from build123d import *

# Parameters (mm, degrees)
SKETCH1_R           = 3.75
SKETCH1_R_2         = 0.65
BOSS_EXTRUDE1_DEPTH = 2.5
CUT_EXTRUDE1_START  = -1.5
SKETCH2_R           = 0.65
CUT_EXTRUDE1_DEPTH  = 1.5
FILLET1_R           = 3
CUT_EXTRUDE3_DEPTH  = 56.730615831
FILLET2_R           = 1.5


with BuildPart() as part:
    # Sketch1 → Boss-Extrude1 (new body)
    with BuildSketch(Plane(origin=(0, 0, 0), x_dir=(1, 0, 0), z_dir=(0, 1, 0))):
        Polygon((0, 0), (0, 12), (50, 25.397459622), (50, 0), align=None)
        with Locations(Location((5.75, 6, 0), (0, 0, 270))):
            Circle(SKETCH1_R, mode=Mode.SUBTRACT)
        with Locations(Location((22.75, 6, 0), (0, 0, 270))):
            Circle(SKETCH1_R_2, mode=Mode.SUBTRACT)
        with Locations(Location((45.166201183, 17.5, 0), (0, 0, 270))):
            Circle(SKETCH1_R, mode=Mode.SUBTRACT)
        with Locations(Location((36.666201183, 2.777568136, 0), (0, 0, 270))):
            Circle(SKETCH1_R_2, mode=Mode.SUBTRACT)
        with Locations(Location((37.916201183, 4.942631645, 0), (0, 0, 270))):
            Circle(SKETCH1_R_2, mode=Mode.SUBTRACT)
        with Locations(Location((39.166201183, 7.107695155, 0), (0, 0, 270))):
            Circle(SKETCH1_R_2, mode=Mode.SUBTRACT)
        with Locations(Location((40.416201183, 9.272758664, 0), (0, 0, 270))):
            Circle(SKETCH1_R_2, mode=Mode.SUBTRACT)
        with Locations(Location((41.666201183, 11.437822174, 0), (0, 0, 270))):
            Circle(SKETCH1_R_2, mode=Mode.SUBTRACT)
        with Locations(Location((20.25, 6, 0), (0, 0, 270))):
            Circle(SKETCH1_R_2, mode=Mode.SUBTRACT)
        with Locations(Location((17.75, 6, 0), (0, 0, 270))):
            Circle(SKETCH1_R_2, mode=Mode.SUBTRACT)
        with Locations(Location((15.25, 6, 0), (0, 0, 270))):
            Circle(SKETCH1_R_2, mode=Mode.SUBTRACT)
        with Locations(Location((12.75, 6, 0), (0, 0, 270))):
            Circle(SKETCH1_R_2, mode=Mode.SUBTRACT)
    extrude(amount=BOSS_EXTRUDE1_DEPTH)

    # Sketch2 → Cut-Extrude1 (cut)
    # profile 1 of 3: a face of its own
    with BuildSketch(Plane(origin=(0, 2.5, 0), x_dir=(1, 0, 0), z_dir=(0, 1, 0)).offset(CUT_EXTRUDE1_START)):
        with BuildLine():
            Line((22.25, 8.5), (6.610232527, 9.65))
            ThreePointArc((6.610232527, 9.65), (8.690099656, 8.32772722), (9.5, 6))
            ThreePointArc((9.5, 6), (8.690099656, 3.67227278), (6.610232527, 2.35))
            Line((6.610232527, 2.35), (22.25, 3.5))
            ThreePointArc((22.25, 3.5), (24.75, 6), (22.25, 8.5))
        make_face()
        with Locations(Location((12.75, 6, 0), (0, 0, 270))):
            Circle(SKETCH2_R, mode=Mode.SUBTRACT)
        with Locations(Location((15.25, 6, 0), (0, 0, 270))):
            Circle(SKETCH2_R, mode=Mode.SUBTRACT)
        with Locations(Location((17.75, 6, 0), (0, 0, 270))):
            Circle(SKETCH2_R, mode=Mode.SUBTRACT)
        with Locations(Location((20.25, 6, 0), (0, 0, 270))):
            Circle(SKETCH2_R, mode=Mode.SUBTRACT)
        with Locations(Location((22.75, 6, 0), (0, 0, 270))):
            Circle(SKETCH2_R, mode=Mode.SUBTRACT)
    # profile 2 of 3: a face of its own
    with BuildSketch(Plane(origin=(0, 2.5, 0), x_dir=(1, 0, 0), z_dir=(0, 1, 0)).offset(CUT_EXTRUDE1_START)):
        with BuildLine():
            ThreePointArc((47.897077643, 14.930016779), (45.712022261, 13.789935398), (43.291201183, 14.252404736))
            Line((43.291201183, 14.252404736), (41.991201183, 12.000738686))
            ThreePointArc((41.991201183, 12.000738686), (42.229117695, 11.762822174), (42.316201183, 11.437822174))
            ThreePointArc((42.316201183, 11.437822174), (41.991201183, 10.874905661), (41.341201183, 10.874905661))
            Line((41.341201183, 10.874905661), (40.741201183, 9.835675177))
            ThreePointArc((40.741201183, 9.835675177), (40.979117695, 9.597758664), (41.066201183, 9.272758664))
            ThreePointArc((41.066201183, 9.272758664), (40.741201183, 8.709842152), (40.091201183, 8.709842152))
            Line((40.091201183, 8.709842152), (39.491201183, 7.670611667))
            ThreePointArc((39.491201183, 7.670611667), (39.729117695, 7.432695155), (39.816201183, 7.107695155))
            ThreePointArc((39.816201183, 7.107695155), (39.491201183, 6.544778642), (38.841201183, 6.544778642))
            Line((38.841201183, 6.544778642), (38.241201183, 5.505548158))
            ThreePointArc((38.241201183, 5.505548158), (38.479117695, 5.267631645), (38.566201183, 4.942631645))
            ThreePointArc((38.566201183, 4.942631645), (38.241201183, 4.379715133), (37.591201183, 4.379715133))
            Line((37.591201183, 4.379715133), (36.991201183, 3.340484648))
            ThreePointArc((36.991201183, 3.340484648), (37.229117695, 3.102568136), (37.316201183, 2.777568136))
            ThreePointArc((37.316201183, 2.777568136), (36.991201183, 2.214651623), (36.341201183, 2.214651623))
            Line((36.341201183, 2.214651623), (35.666201183, 1.045517328))
            ThreePointArc((35.666201183, 1.045517328), (37.563248796, 0.795766272), (39.081264692, 1.960580838))
            Line((39.081264692, 1.960580838), (47.897077643, 14.930016779))
        make_face()
    # profile 3 of 3: a face of its own
    with BuildSketch(Plane(origin=(0, 2.5, 0), x_dir=(1, 0, 0), z_dir=(0, 1, 0)).offset(CUT_EXTRUDE1_START)):
        with BuildLine():
            Line((41.991201183, 12.000738686), (43.291201183, 14.252404736))
            ThreePointArc((43.291201183, 14.252404736), (41.680280449, 16.117662618), (41.575092196, 18.580016779))
            Line((41.575092196, 18.580016779), (34.751137673, 4.460580838))
            ThreePointArc((34.751137673, 4.460580838), (34.501386617, 2.563533225), (35.666201183, 1.045517328))
            Line((35.666201183, 1.045517328), (36.341201183, 2.214651623))
            ThreePointArc((36.341201183, 2.214651623), (36.10328467, 3.102568136), (36.991201183, 3.340484648))
            Line((36.991201183, 3.340484648), (37.591201183, 4.379715133))
            ThreePointArc((37.591201183, 4.379715133), (37.35328467, 5.267631645), (38.241201183, 5.505548158))
            Line((38.241201183, 5.505548158), (38.841201183, 6.544778642))
            ThreePointArc((38.841201183, 6.544778642), (38.60328467, 7.432695155), (39.491201183, 7.670611667))
            Line((39.491201183, 7.670611667), (40.091201183, 8.709842152))
            ThreePointArc((40.091201183, 8.709842152), (39.85328467, 9.597758664), (40.741201183, 9.835675177))
            Line((40.741201183, 9.835675177), (41.341201183, 10.874905661))
            ThreePointArc((41.341201183, 10.874905661), (41.10328467, 11.762822174), (41.991201183, 12.000738686))
        make_face()
    extrude(amount=CUT_EXTRUDE1_DEPTH, mode=Mode.SUBTRACT)

    # Fillet1
    fillet1_edges = [part.edges().sort_by_distance(p)[0] for p in [
        (50, 1.25, 0),
        (0, 1.25, 0),
        (0, 1.25, -12),
        (50, 1.25, -25.397459622),
    ]]
    fillet(fillet1_edges, radius=FILLET1_R)

    # Sketch3 → Cut-Extrude3 (cut, through all)
    with BuildSketch(Plane(origin=(0, 2.5, 0), x_dir=(1, 0, 0), z_dir=(0, 1, 0))):
        Polygon((18.580286951, 13.872744342), (39.830655129, 19.566763335), (31.823901882, 3), align=None)
    extrude(amount=-CUT_EXTRUDE3_DEPTH, mode=Mode.SUBTRACT)

    # Fillet2
    fillet2_edges = [part.edges().sort_by_distance(p)[0] for p in [
        (31.823901882, 1.25, -3),
        (18.580286951, 1.25, -13.872744342),
        (39.830655129, 1.25, -19.566763335),
    ]]
    fillet(fillet2_edges, radius=FILLET2_R)


solid = part.part
Part model, mm, in its own coordinate system. A direction names the side the tool comes from. Give positions to 0.01 mm unless a question says otherwise; leave off trailing zeros. Order: outer loops, then holes, each group sorted by start corner. A loop starts at its lowest first (then second) coordinate and runs counter-clockwise, first axis right, second up. Notation, with made-up numbers: (23.25, -7.75) - (31.25, -7.75) arc R27 ccw to (31.25, 8.25) - close; hole circle Ø11 at (-36.5, -8.75). An arc over 180 degrees is marked (long way). Use a Markdown table: item, result.
1) Saw through at D-D on x = 5.75. List the corners of the cut face in (y, z), plus the area to 3 significant figures.
Checked values:
| item | result |
|---|---|
| outline | (0, -13.54) - (2.5, -13.54) - (2.5, -9.75) - (0, -9.75) - close; (0, -2.25) - (2.5, -2.25) - (2.5, 0) - (0, 0) - close |
| area | 15.1 mm² |
2) Two-plate mould, pull along Z, no slides. Class faces 1 (the cylindrical face through (24.75, 1.74, -5.95)), 2 (the flat face through (25, 1, 0)), 3 (the flat face through (0, 1, -6)): +Z half, -Z half, draft (parallel to the pull), parting line (faces both ways), or undercut.
Checked values:
| item | result |
|---|---|
| face 1 | undercut |
| face 2 | +Z half |
| face 3 | draft |
3) Flat gauge pin, fed straight in: P1, Ø1.7, axis at x = 39.17, z = -7.11, coming from the +Y side. Where does the tip first touch, or does it go through?
Checked values:
| item | result |
|---|---|
| P1 | y = 1 |
4) Saw through at C-C on x = 26. List the corners of the cut face in (y, z).
Checked values:
| item | result |
|---|---|
| outline | (0, -18.97) - (2.5, -18.97) - (2.5, -15.86) - (0, -15.86) - close; (0, -7.78) - (2.5, -7.78) - (2.5, 0) - (0, 0) - close |
5) 3-axis set-ups, long thin cutter, end or side, ignore diameter. For faces 4 (the cylindrical face through (0.86, 1.27, -0.9)), 5 (the flat face through (43.427, 1.74, -8.355)), 6 (the cylindrical face through (20.318, 1.232, -13.474)): which of +Z, -Z, +X, -X, +Y, -Y reach the whole face in a straight line?
Checked values:
| item | result |
|---|---|
| face 4 | +Z, -X, +Y, -Y |
| face 5 | +Y |
| face 6 | +Y, -Y |
6) Saw through at B-B on z = -17.5. List the corners of the cut face in (x, y).
Checked values:
| item | result |
|---|---|
| outline | (20.53, 0) - (32.12, 0) - (32.12, 2.5) - (20.53, 2.5) - close; (38.54, 0) - (41.42, 0) - (41.42, 1) - (41.05, 1) - (41.05, 2.5) - (38.54, 2.5) - close; (48.92, 0) - (50, 0) - (50, 2.5) - (48.92, 2.5) - close |
7) Probe L1, parallel to X at y = 1.75, z = -12; L2, parallel to X at y = 0.75, z = -12; L3, parallel to Z at x = 47, y = 0.95. List the from-to ranges inside material, lowest first. Write a range as from..to.
Checked values:
| item | result |
|---|---|
| L1 | 1.08..20.86, 36.17..38.39, 45.91..50 |
| L2 | 1.08..20.86, 36.17..41.34, 41.99..50 |
| L3 | -24.49..-20.77, -14.23..0 |
8) Saw through at A-A on y = 1.6. List the corners of the cut face in (x, z).
Checked values:
| item | result |
|---|---|
| outline | (0, -9.7) arc R3 ccw to (2.22, -12.6) - (46.22, -24.39) arc R3 ccw to (50, -21.49) - (50, -3) arc R3 ccw to (47, 0) - (3, 0) arc R3 ccw to (0, -3) - close; hole (6.61, -9.65) - (22.25, -8.5) arc R2.5 ccw to (22.25, -3.5) - (6.61, -2.35) arc R3.75 ccw (long way) to start; hole (20.84, -12.02) arc R1.5 ccw to (21.4, -14.63) - (36.67, -18.72) arc R1.5 ccw to (38.41, -16.62) - (32.65, -4.72) arc R1.5 ccw to (30.35, -4.21) - close; hole (34.75, -4.46) - (41.58, -18.58) arc R3.75 ccw (long way) to (47.9, -14.93) - (39.08, -1.96) arc R2.5 ccw to start |
